Verification items for this drawing (mm, ordinates from the low corner). Round coordinates to 2 decimals unless told otherwise and drop trailing zeros. Order: outer loops, then holes, each group sorted by start corner. A loop starts at its lowest first (then second) coordinate and runs counter-clockwise, first axis right, second up. Notation, with made-up numbers: (-35.75, 73) - (-20.75, 73) arc R29 ccw to (-20.75, 112) - close; hole circle Ø2 at (69.25, 80). An arc over 180 degrees is marked (long way). Return JSON: item names as keys, results as strings. Group by question number.
Q1. Sectioned sample at D-D, the plane z = 50. Record the cut outline in (x, y).
Q2. Sectioned sample at A-A, the plane z = 23.5. Record the cut outline in (x, y) (1 decimal).
Q3. Sectioned sample at B-B, the plane y = 0.8. Record the cut outline in (x, z).
Q4. Material ranges on line 1 along X through (y, z) = (0.6, 72) (1 decimal); line 2 along X through (y, z) = (0.6, 82); line 3 along Z through (x, y) = (67, 0.6) (1 decimal), recorded low to high.
Q5. Sectioned sample at C-C, the plane x = 18. Record the cut outline in (y, z).
Q6. Gauge pin test, flat end, axial feed: pin 1 Ø0.5 at (y, z) = (0.5, 84) entering from -X. Record the tip position at first contact, or that the pin passes through.
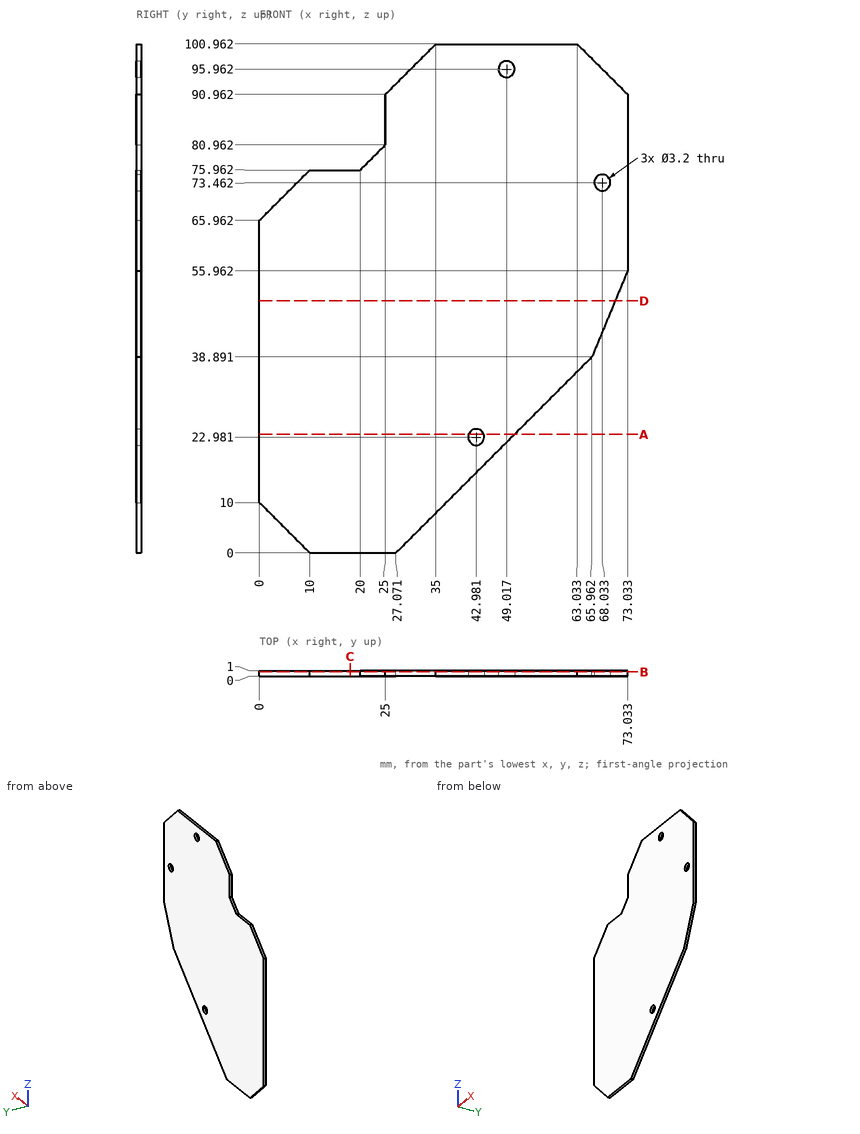
Reply:
{
 "1": {"outline": "(0, 0) - (70.56, 0) - (70.56, 1) - (0, 1) - close"},
 "2": {"outline": "(0, 0) - (41.5, 0) - (41.5, 1) - (0, 1) - close; (44.5, 0) - (50.6, 0) - (50.6, 1) - (44.5, 1) - close"},
 "3": {"outline": "(0, 10) - (10, 0) - (27.07, 0) - (65.96, 38.89) - (73.03, 55.96) - (73.03, 90.96) - (63.03, 100.96) - (35, 100.96) - (25, 90.96) - (25, 80.96) - (20, 75.96) - (10, 75.96) - (0, 65.96) - close; hole circle Ø3.2 at (42.98, 22.98); hole circle Ø3.2 at (49.02, 95.96); hole circle Ø3.2 at (68.03, 73.46)"},
 "4": {"line 1": "6 to 67.4, 68.7 to 73", "line 2": "25 to 73.03", "line 3": "41.4 to 72.2, 74.7 to 97"},
 "5": {"outline": "(0, 0) - (1, 0) - (1, 75.96) - (0, 75.96) - close"},
 "6": {"pin 1": "x = 25"}
}
